from build123d import *

# Parameters (mm, degrees)
SKETCH1_W           = 100
SKETCH1_H           = 46.3
SKETCH1_R           = 1.5
SKETCH1_R_2         = 8
BOSS_EXTRUDE1_DEPTH = 5


with BuildPart() as part:
    # Sketch1 → Boss-Extrude1 (new body)
    with BuildSketch(Plane.XY):
        Rectangle(SKETCH1_W, SKETCH1_H)
        with Locations(Location((46, 19.15, 0), (0, 0, 180))):
            Circle(SKETCH1_R, mode=Mode.SUBTRACT)
        with Locations((-46, 19.15)):
            Circle(SKETCH1_R, mode=Mode.SUBTRACT)
        with Locations((46, -19.15)):
            Circle(SKETCH1_R, mode=Mode.SUBTRACT)
        with Locations(Location((-46, -19.15, 0), (0, 0, 180))):
            Circle(SKETCH1_R, mode=Mode.SUBTRACT)
        with Locations((-30.5, 0)):
            Circle(SKETCH1_R_2, mode=Mode.SUBTRACT)
    extrude(amount=BOSS_EXTRUDE1_DEPTH)


solid = part.part
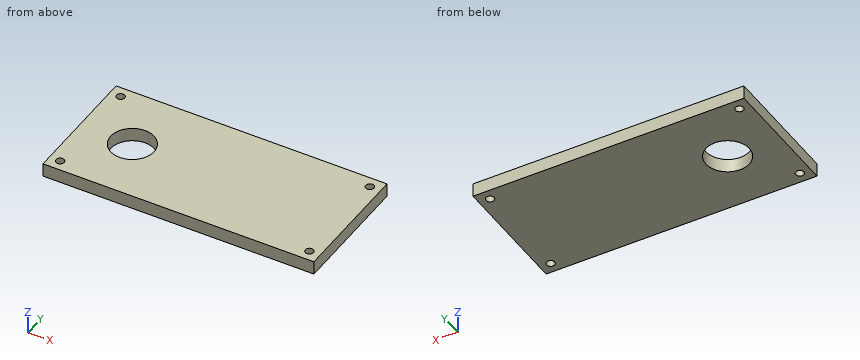
Here's how the part is built. I have some questions about the finished solid (model axes, mm). Round coordinates to 2 decimals unless told otherwise and drop trailing zeros. Write each loop counter-clockwise with the first axis right and the second up, starting at its lowest first coordinate (ties: lowest second). Pieces come first, ordered by that corner, then holes.
1. I need wall thicknesses on L1, parallel to Y at x = 46, z = 2.15; L2, parallel to X at y = -18, z = 3.7; L3, parallel to X at y = -1.5, z = 3. Which ranges of each line are inside material? Lowest first, please.
2. Suppose I cut it at A-A (z = 4.2). List the corners of the cut face in (x, y) for me, and give its area (3 significant figures).
3. Suppose I cut it at C-C (x = -30.5). List the corners of the cut face in (y, z) for me.
4. Suppose I cut it at B-B (y = 0). List the corners of the cut face in (x, z) for me.
5. Suppose I cut it at D-D (x = 46). List the corners of the cut face in (y, z) for me.
Answer sheet:
1. L1: y = -23.15 to -20.65, -17.65 to 17.65, 20.65 to 23.15
1. L2: x = -50 to -46.96, -45.04 to 45.04, 46.96 to 50
1. L3: x = -50 to -38.36, -22.64 to 50
2. outline: (-50, -23.15) - (50, -23.15) - (50, 23.15) - (-50, 23.15) - close; hole circle Ø3 at (-46, -19.15); hole circle Ø3 at (-46, 19.15); hole circle Ø16 at (-30.5, 0); hole circle Ø3 at (46, -19.15); hole circle Ø3 at (46, 19.15)
2. area: 4,400 mm2
3. outline: (-23.15, 0) - (-8, 0) - (-8, 5) - (-23.15, 5) - close; (8, 0) - (23.15, 0) - (23.15, 5) - (8, 5) - close
4. outline: (-50, 0) - (-38.5, 0) - (-38.5, 5) - (-50, 5) - close; (-22.5, 0) - (50, 0) - (50, 5) - (-22.5, 5) - close
5. outline: (-23.15, 0) - (-20.65, 0) - (-20.65, 5) - (-23.15, 5) - close; (-17.65, 0) - (17.65, 0) - (17.65, 5) - (-17.65, 5) - close; (20.65, 0) - (23.15, 0) - (23.15, 5) - (20.65, 5) - close
